Geometry: see drawing. Coordinates: mm, zero at the bounding-box minimum. Give positions to 0.01 mm unless a question says otherwise; leave off trailing zeros. Loops run counter-clockwise (first coordinate to the right, second up) from the corner with the lowest first, then second, coordinate; pieces in that order, holes last. Notation, with made-up numbers: M 14.25,-11.75 L 33.25,-11.75 A27 cw 33.25,13.25 Z; hole C -37,-33.5 d2. An arc over 180 degrees is marked long. Use a Markdown table: item, result. Add a question column.
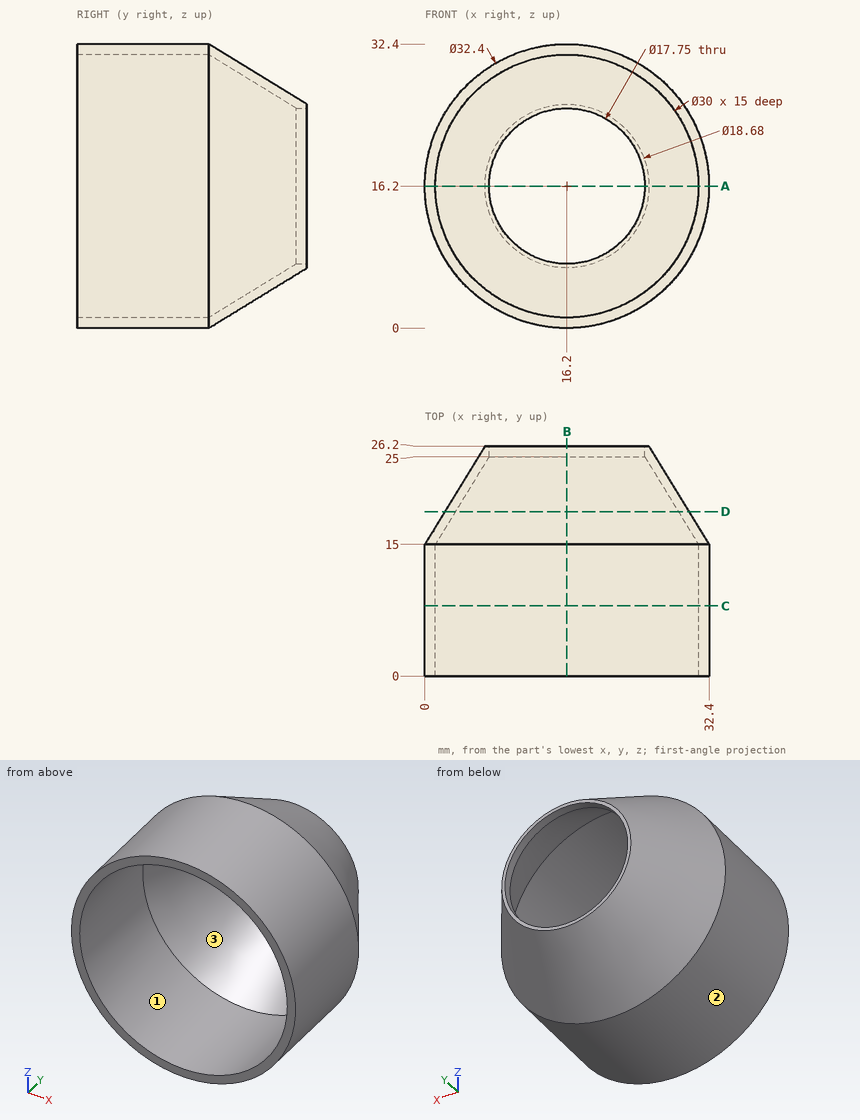
1) Ray query, line 1 (X direction, y = 9.5, z = 16.2); line 2 (X direction, y = 9, z = 12.5). Return the intervals inside material, ascending. Write a range as [from, to].
2) Section query A-A, the plane z = 16.2. Return the cut outline in (x, y) (3 decimals), and give its area (3 significant figures).
3) Contact query for flat-ended pins moving along their axis: P1, Ø8, axis at y = 11, z = 16, coming from the -X side; P2, Ø16, axis at x = 16.2, z = 16.2, coming from the +Y side; P3, Ø6, axis at y = 8.5, z = 25.5, coming from the -X side; P4, Ø4, axis at x = 20, y = 9, coming from the +Z side. Output: stop coordinate, or through.
4) Section query B-B, the plane x = 16.2. Return the cut outline in (y, z) (3 decimals), and give its area (3 significant figures).
5) Pull-direction query (X, two-part tool) for the marked faces 1, 2 and 3; classes: pulls with the +X half, pulls with the -X half, needs draft (parallel to the pull), parting line crosses it, or undercut.
6) Section query D-D, the plane y = 18.75. Return the cut outline in (x, z), and give its area (3 significant figures).
7) Section query C-C, the plane y = 8. Return the cut outline in (x, z).
Entries:
| question | item | result |
|---|---|---|
| 1 | line 1 | x = [0, 1.2], [31.2, 32.4] |
| 1 | line 2 | x = [0.43, 1.66], [30.74, 31.97] |
| 2 | outline | M 0,0 L 1.2,0 L 1.2,15 L 7.325,25 L 7.325,26.2 L 6.86,26.2 L 0,15 Z; M 25.075,25 L 31.2,15 L 31.2,0 L 32.4,0 L 32.4,15 L 25.54,26.2 L 25.075,26.2 Z |
| 2 | area | 62.0 mm² |
| 3 | P1 | stops at x = 0 |
| 3 | P2 | passes through |
| 3 | P3 | stops at x = 1.28 |
| 3 | P4 | stops at z = 32.3 |
| 4 | outline | M 0,0 L 15,0 L 26.2,6.86 L 26.2,7.325 L 25,7.325 L 15,1.2 L 0,1.2 Z; M 0,31.2 L 15,31.2 L 25,25.075 L 26.2,25.075 L 26.2,25.54 L 15,32.4 L 0,32.4 Z |
| 4 | area | 62.0 mm² |
| 5 | face 1 | undercut |
| 5 | face 2 | parting line crosses it |
| 5 | face 3 | undercut |
| 6 | outline | C 16.2,16.2 d27.81; hole C 16.2,16.2 d25.41 |
| 6 | area | 100 mm² |
| 7 | outline | C 16.2,16.2 d32.4; hole C 16.2,16.2 d30 |
